Check sheet for the drawn part. Datum: minimum x, y, z corner. Units: mm. A direction names the side the tool comes from. Round coordinates to 2 decimals unless told otherwise and drop trailing zeros. Write each loop counter-clockwise with the first axis right and the second up, starting at its lowest first coordinate (ties: lowest second). Pieces come first, ordered by that corner, then holes. Notation, with made-up numbers: (69, 86) - (94, 86) arc R12 ccw to (94, 98) - close; hole circle Ø11 at (12, 50.25). An arc over 180 degrees is marked (long way). Answer as a JSON object with one key per item and string values. Group by question number.
Item 1: Set-up check for the marked faces 1, 2 and 3: record each of +Z, -Z, +X, -X, +Y, -Y from which the full face is reachable in a straight line by a thin tool's end or side.
Item 2: Sectioned sample at A-A on z = 35. Record the boundary of the cut face in (x, y).
Item 3: Sectioned sample at D-D on z = 15. Record the boundary of the cut face in (x, y).
Item 4: Sectioned sample at C-C on y = 40. Record the boundary of the cut face in (x, z).
Item 5: Sectioned sample at B-B on x = 30. Record the boundary of the cut face in (y, z), plus the area to 3 significant figures.
Item 6: Release check for a two-part mould opening along Z. For the marked faces 4, 5 and 6 record: pulls with the +Z half, pulls with the -Z half, needs draft (parallel to the pull), parting line crosses it, or undercut.
Item 7: Thickness scan on line 1 (X direction, y = 10.5, z = 35); line 2 (Z direction, x = 38, y = 43); line 3 (Z direction, x = 56.5, y = 55.5). Record the ranges inside material, lowest first.
Item 8: Gauge pin test, flat ends, axial feed: P1, Ø10, axis at x = 53, z = 38, coming from the +Y side; P2, Ø1.5, axis at x = 40, y = 35.5, coming from the -Z side; P3, Ø1.5, axis at y = 36, z = 52.5, coming from the +X side. Record the tip position at first contact, or that the pin passes through.
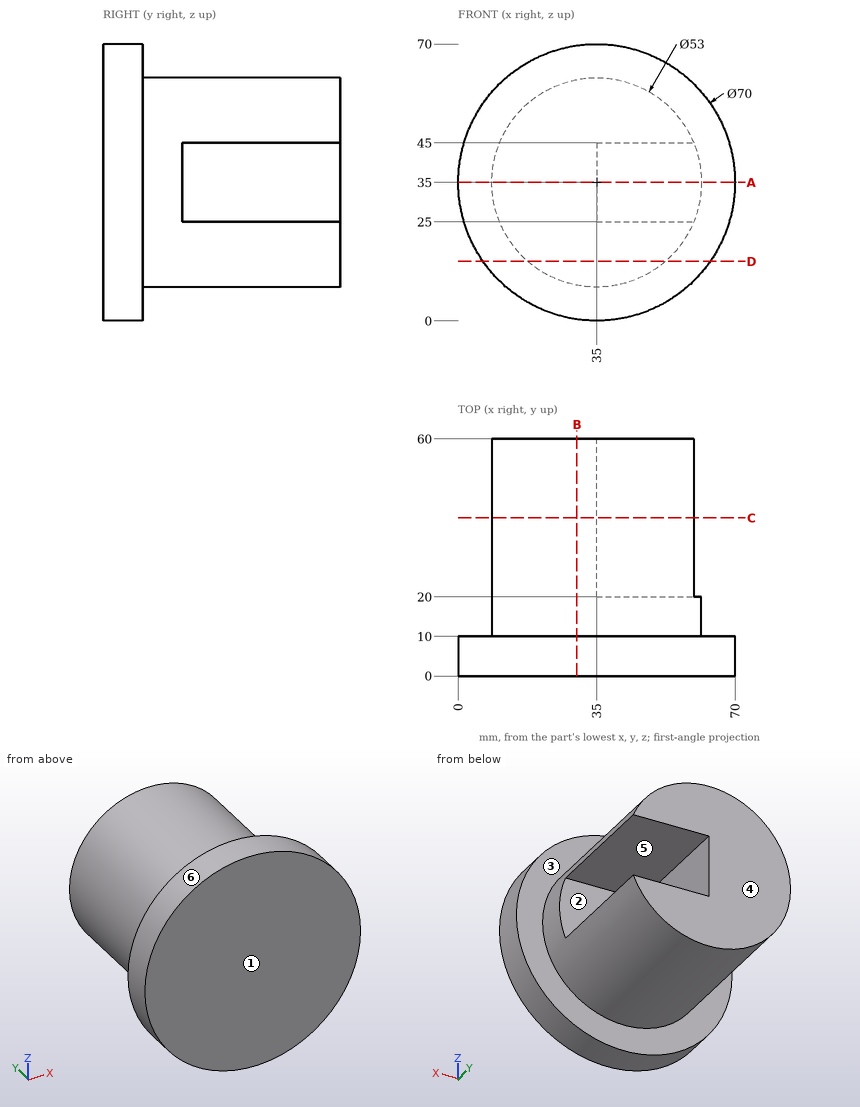
Completed:
{
 "1": {"face 1": "+Z, -Z, +X, -X, -Y", "face 2": "+X, +Y", "face 3": "+Y"},
 "2": {"outline": "(0, 0) - (70, 0) - (70, 10) - (61.5, 10) - (61.5, 20) - (35, 20) - (35, 60) - (8.5, 60) - (8.5, 10) - (0, 10) - close"},
 "3": {"outline": "(6.28, 0) - (63.72, 0) - (63.72, 10) - (52.39, 10) - (52.39, 60) - (17.61, 60) - (17.61, 10) - (6.28, 10) - close"},
 "4": {"outline": "(35, 25) - (35, 45) - (59.54, 45) arc R26.5 ccw (long way) to (59.54, 25) - close"},
 "5": {"outline": "(0, 0.36) - (10, 0.36) - (10, 8.98) - (60, 8.98) - (60, 61.02) - (10, 61.02) - (10, 69.64) - (0, 69.64) - close", "area": "3,300 mm²"},
 "6": {"face 4": "needs draft", "face 5": "undercut", "face 6": "parting line crosses it"},
 "7": {"line 1": "8.5 to 61.5", "line 2": "8.67 to 25, 45 to 61.33", "line 3": "19.51 to 25, 45 to 50.49"},
 "8": {"P1": "y = 20", "P2": "z = 8.84", "P3": "x = 55.54"}
}
